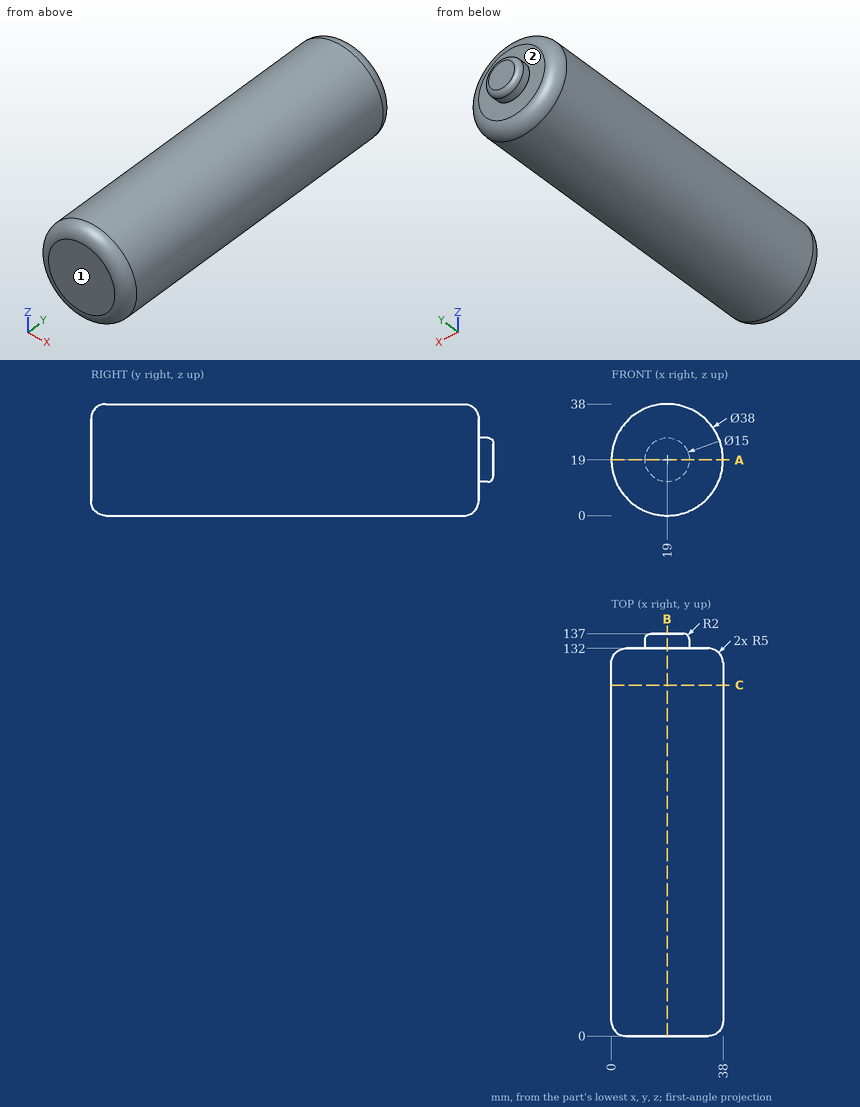
Verification items for this drawing (mm, ordinates from the low corner). A direction names the side the tool comes from. Round coordinates to 2 decimals unless told otherwise and drop trailing zeros. Write each loop counter-clockwise with the first axis right and the second up, starting at its lowest first coordinate (ties: lowest second). Pieces come first, ordered by that corner, then holes. Notation, with made-up numbers: M 89.25,-31.75 L 145.25,-31.75 A19 ccw 145.25,5.25 Z; hole C 72.5,16 d3. An arc over 180 degrees is marked long. Write item = value, one per line. Start each with the question number.
1. Section check C-C, the plane y = 119.5. Record the cut outline in (x, z), then the cut area to 3 significant figures.
2. Gauge pin test, flat ends, axial feed: pin 1 (2 mm diameter, centred on x = 9.5, z = 22, fed in from +Y); pin 2 (1.5 mm diameter, centred on y = 57, z = 23, fed in from -X); pin 3 (12 mm diameter, centred on x = 5.5, y = 32.5, fed in from -Z). Record the tip position at first contact, or that the pin passes through.
3. Scan lines: line 1 (X direction, y = 74.5, z = 20); line 2 (Y direction, x = 24, z = 22); line 3 (Z direction, x = 19.5, y = 58). Record each from-to range of solid material in increasing order. Write a range as [from, to].
4. Section check A-A, the plane z = 19. Record the cut outline in (x, y).
5. Section check B-B, the plane x = 19. Record the cut outline in (y, z), then the cut area to 3 significant figures.
6. Tool access check on the marked faces 1 and 2. Record the directions out of +Z, -Z, +X, -X, +Y, -Y that give a thin tool (end or side, any length) a straight path to the whole face; none if there is none.
Results found:
q1.outline = C 19,19 d38
q1.area = 1,130 mm^2
q2.pin_1 = 132
q2.pin_2 = 0.28
q2.pin_3 = 1.54
q3.line_1 = [0.03, 37.97]
q3.line_2 = [0, 136.97]
q3.line_3 = [0.01, 37.99]
q4.outline = M 0,5 A5 ccw 5,0 L 33,0 A5 ccw 38,5 L 38,127 A5 ccw 33,132 L 26.5,132 L 26.5,135 A2 ccw 24.5,137 L 13.5,137 A2 ccw 11.5,135 L 11.5,132 L 5,132 A5 ccw 0,127 Z
q5.outline = M 0,5 A5 ccw 5,0 L 127,0 A5 ccw 132,5 L 132,11.5 L 135,11.5 A2 ccw 137,13.5 L 137,24.5 A2 ccw 135,26.5 L 132,26.5 L 132,33 A5 ccw 127,38 L 5,38 A5 ccw 0,33 Z
q5.area = 5,070 mm^2
q6.face_1 = +Z, -Z, +X, -X, -Y
q6.face_2 = +Y
